Here's how the part is built. I have some questions about the finished solid (model axes, mm). A direction names the side the tool comes from. Round coordinates to 2 decimals unless told otherwise and drop trailing zeros. Loops run counter-clockwise (first coordinate to the right, second up) from the corner with the lowest first, then second, coordinate; pieces in that order, holes last. Notation, with made-up numbers: M 51,-25.5 L 63,-25.5 A7 cw 63,-17.5 Z; hole C 43.25,-37.5 d6. An arc over 180 degrees is marked long. Answer as CSV lines item,"result".
```python
from build123d import *

# Parameters (mm, degrees)
F0_W     = 44
F0_H     = 74
F1_DEPTH = 5
F2_W     = 5
F2_H     = 27
F3_DEPTH = 238
F0_W_2   = 40
F0_H_2   = 70
F4_DEPTH = 35
F5_R     = 4.99999


# Not quite as in the source:
# - a fillet or chamfer is up to 0.001 mm smaller than in the source, because OpenCascade refuses the exact size


with BuildPart() as f1:
    # F0 (on Top) → F1 (new body)
    with BuildSketch(Plane.XY):
        Polygon((106.4276799491, 10), (-131.5723200509, 10), (-131.5723200509, -80), (-129.5723200509, -80), (106.4276799491, -80), align=None)
        with Locations((-102.5723200509, -35)):
            Rectangle(F0_W, F0_H, mode=Mode.SUBTRACT)
        with Locations((-42.5723200509, -35)):
            Rectangle(F0_W, F0_H, mode=Mode.SUBTRACT)
        with Locations((17.4276799491, -35)):
            Rectangle(F0_W, F0_H, mode=Mode.SUBTRACT)
        with Locations((77.4276799491, -35)):
            Rectangle(F0_W, F0_H, mode=Mode.SUBTRACT)
    extrude(amount=F1_DEPTH)

    # F2 (on face) → F3 (join)
    with BuildSketch(Plane(origin=(-131.5723200509, 0, 0), x_dir=(0, -1, 0), z_dir=(-1, 0, 0))):
        Polygon((120, 32), (120, 37), (75, 37), (75, 32), (80, 32), align=None)
        with Locations((77.5, 18.5)):
            Rectangle(F2_W, F2_H)
    extrude(amount=-F3_DEPTH)

    # F0 (on Top) → F4 (join)
    with BuildSketch(Plane.XY):
        with Locations((-102.5723200509, -35)):
            Rectangle(F0_W, F0_H)
        with Locations((-102.5723200509, -35)):
            Rectangle(F0_W_2, F0_H_2, mode=Mode.SUBTRACT)
        with Locations((-42.5723200509, -35)):
            Rectangle(F0_W, F0_H)
        with Locations((-42.5723200509, -35)):
            Rectangle(F0_W_2, F0_H_2, mode=Mode.SUBTRACT)
        with Locations((17.4276799491, -35)):
            Rectangle(F0_W, F0_H)
        with Locations((17.4276799491, -35)):
            Rectangle(F0_W_2, F0_H_2, mode=Mode.SUBTRACT)
        with Locations((77.4276799491, -35)):
            Rectangle(F0_W, F0_H)
        with Locations((77.4276799491, -35)):
            Rectangle(F0_W_2, F0_H_2, mode=Mode.SUBTRACT)
    extrude(amount=F4_DEPTH)

    # F5 (radius 5 in the source; OpenCascade refuses exactly that, so slightly less here)
    f5_edges = [f1.edges().sort_by_distance(p)[0] for p in [
        (-12.57232, 10, 0),
        (-131.57232, -35, 0),
        (106.42768, -35, 0),
        (106.42768, 10, 2.5),
        (-131.57232, 10, 2.5),
    ]]
    fillet(f5_edges, radius=F5_R)


solid = f1.part
```
1. I want a section at B-B, the plane z = 15. Count the separate pieces of the cut face and the enclosed holes in it, and give its area (3 significant figures).
Evaluation:
separate pieces,"5"
enclosed holes,"4"
area,"3,010 mm²"
2. Which directions (+Z, -Z, +X, -X, +Y, -Y) give clear straight access to the entire face, cutting with the end or side of a thin tool? Please do faces 5 (the flat face through (17, 2, 20)), 6 (the flat face through (77, -72, 20)), 7 (the cylindrical face through (-14, 9, 2)), 8 (the flat face through (-14, -100, 32)), 9 (the flat face through (37.428, -35, 17)).
Evaluation:
face 5,"+Z, +X, -X, +Y"
face 6,"+Z, +X, -X"
face 7,"-Z, +X, -X, +Y"
face 8,"-Z, +X, -X, -Y"
face 9,"+Z, -Z"
3. For P1, Ø10.5, axis at y = -31, z = 23.5, coming from the -X side; P2, Ø4, axis at x = -58.5, y = -93, coming from the -Z side; P3, Ø15, axis at x = 23.5, z = 20, coming from the +Y side, each with a flat end and sliding along its axis, tell me the tip position at first contact or that it passes through.
Evaluation:
P1,"stops at x = -124.57"
P2,"stops at z = 32"
P3,"stops at y = 2"
4. I want a section at D-D, the plane y = -106. Please give me the cut outline in (x, z), and give its area (3 significant figures).
Evaluation:
outline,"M -131.57,32 L 106.43,32 L 106.43,37 L -131.57,37 Z"
area,"1,190 mm²"
5. If I drill on line 1 (Y direction, x = -60.5, z = 6.5); line 2 (Y direction, x = -51.5, z = 34); line 3 (Z direction, x = 79, y = -103), over which ranges is the centre line in solid material (lowest first)? Write a range as [from, to].
Evaluation:
line 1,"y = [-80, -75], [-72, -70], [0, 2]"
line 2,"y = [-120, -75], [-72, -70], [0, 2]"
line 3,"z = [32, 37]"
6. We'd pull the mould along Y, two halves only. Please class faces 1 (the flat face through (77, -70, 17)), 2 (the flat face through (-122.572, -35, 17)), 3 (the flat face through (-14, -80, 16)), 4 (the flat face through (-124.572, -36, 20)): pulls with the +Y half, pulls with the -Y half, needs draft (parallel to the pull), parting line crosses it, or undercut.
Evaluation:
face 1,"undercut"
face 2,"undercut"
face 3,"pulls with the -Y half"
face 4,"needs draft"
